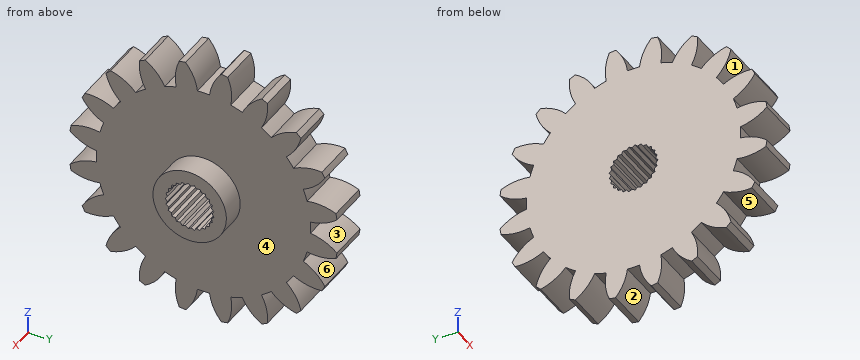
from build123d import *

# Parameters (mm, degrees)
BASPROSKE_W         = 5
BASPROSKE_H         = 16.5
TOOTHCUT_DEPTH      = 24.864199128
TEETHCUTS_COUNT     = 20
TEETHCUTS_ANGLE     = 342
BORSKE_R            = 2.5
BORE_DEPTH          = 50.0000508
BOSS_EXTRUDE1_START = 3
SKETCH1_R           = 4.5
SKETCH1_R_2         = 2.5
BOSS_EXTRUDE1_DEPTH = 3
SKETCH2_R           = 2.75
SKETCH2_R_2         = 2.5
CUT_EXTRUDE1_DEPTH  = 25.472631648
CIRPATTERN1_COUNT   = 25


with BuildPart() as part:
    # BasProSke → Base-Revolve (revolve)
    with BuildSketch(Plane(origin=(0, 0, 0), x_dir=(1, 0, 0), z_dir=(0, 1, 0)), mode=Mode.PRIVATE) as base_revolve_sk:
        with Locations((2.5, 8.25)):
            Rectangle(BASPROSKE_W, BASPROSKE_H)
    revolve(base_revolve_sk.sketch.rotate(Axis((-10, 0, 0), (1, 0, 0)), 180), axis=Axis((-10, 0, 0), (1, 0, 0)))

    # TooCutSke → ToothCut (cut, through all)
    with BuildSketch(Plane(origin=(0, 0, 0), x_dir=(0, 0, -1), z_dir=(1, 0, 0))):
        with BuildLine():
            ThreePointArc((0.74381438, 13.102904875), (0, 13.124), (-0.74381438, 13.102904875))
            ThreePointArc((-0.74381438, 13.102904875), (-1.226473103, 14.852072512), (-2.209965745, 16.376962373))
            ThreePointArc((-2.209965745, 16.376962373), (0, 16.5254), (2.209965745, 16.376962373))
            ThreePointArc((2.209965745, 16.376962373), (1.226473103, 14.852072512), (0.74381438, 13.102904875))
        make_face()
    toothcut = extrude(amount=TOOTHCUT_DEPTH, mode=Mode.SUBTRACT)

    # TeethCuts: ToothCut ×20 about axis
    teethcuts_axis = Axis((-10, 0, 0), (1, 0, 0))
    for i in range(1, TEETHCUTS_COUNT):
        add(toothcut.rotate(teethcuts_axis, i * TEETHCUTS_ANGLE / (TEETHCUTS_COUNT - 1)), mode=Mode.SUBTRACT)

    # BorSke → Bore (cut, symmetric)
    with BuildSketch(Plane(origin=(0, 0, 0), x_dir=(0, 0, -1), z_dir=(1, 0, 0))):
        with Locations(Location((0, 0, 0), (0, 0, 180))):
            Circle(BORSKE_R)
    extrude(amount=BORE_DEPTH, both=True, mode=Mode.SUBTRACT)

    # Sketch1 → Boss-Extrude1 (add)
    with BuildSketch(Plane(origin=(5, 0, 0), x_dir=(0, 0, -1), z_dir=(1, 0, 0)).offset(BOSS_EXTRUDE1_START)):
        with Locations(Location((0, 0, 0), (0, 0, 180))):
            Circle(SKETCH1_R)
        Circle(SKETCH1_R_2, mode=Mode.SUBTRACT)
    extrude(amount=-BOSS_EXTRUDE1_DEPTH)

    # Sketch2 → Cut-Extrude1 (cut, through all)
    # profile 1 of 2: a face of its own
    with BuildSketch(Plane(origin=(8, 0, 0), x_dir=(0, 0, -1), z_dir=(1, 0, 0))):
        with BuildLine():
            ThreePointArc((0.344666392, -2.728315429), (0, -2.75), (-0.344666392, -2.728315429))
            Line((-0.344666392, -2.728315429), (0, -3))
            Line((0, -3), (0.344666392, -2.728315429))
        make_face()
    # profile 2 of 2: a face of its own
    with BuildSketch(Plane(origin=(8, 0, 0), x_dir=(0, 0, -1), z_dir=(1, 0, 0))):
        Circle(SKETCH2_R)
        Circle(SKETCH2_R_2, mode=Mode.SUBTRACT)
    cut_extrude1 = extrude(amount=-CUT_EXTRUDE1_DEPTH, mode=Mode.SUBTRACT)

    # CirPattern1: Cut-Extrude1 ×25 about axis
    cirpattern1_axis = Axis((0, 0, 0), (1, 0, 0))
    for i in range(1, CIRPATTERN1_COUNT):
        add(cut_extrude1.rotate(cirpattern1_axis, i * 360 / CIRPATTERN1_COUNT), mode=Mode.SUBTRACT)


solid = part.part
Here's how the part is built. I have some questions about the finished solid (model axes, mm). Face numbers are marked on the shaded views. A direction names the side the tool comes from. Give positions to 0.01 mm unless a question says otherwise; leave off trailing zeros. Write each loop counter-clockwise with the first axis right and the second up, starting at its lowest first coordinate (ties: lowest second). Pieces come first, ordered by that corner, then holes. Notation, with made-up numbers: (-22.75, -32) -> (-3.75, -32) arc R11 ccw to (-3.75, -22) -> close; hole circle Ø6 at (-36.5, -4). An arc over 180 degrees is marked (long way). Use one line per item in the form item = value. Start each with the question number.
1. If I drill on L1, parallel to Z at x = 3.75, y = 11.5; L2, parallel to Y at x = 1.75, z = 14; L3, parallel to X at y = -8, z = 5, over which ranges is the centre line in solid material (lowest first)?
2. Will these pins go through, and if not, where does the flat tip stop? pin 1 Ø3 at (y, z) = (-4.5, 8.5) entering from +X; pin 2 Ø10 at (y, z) = (-1, -5.5) entering from +X; pin 3 Ø3 at (x, z) = (2, -6) entering from -Y; pin 4 Ø1 at (x, y) = (4.5, -10.5) entering from -Z.
3. Imagine slicing it at A-A on y = 13.5. List the corners of the cut face in (x, z) for me, plus the area to 3 significant figures.
4. On a 3-axis mill with a long thin cutter (end or side, diameter ignored), from which of +Z, -Z, +X, -X, +Y, -Y can I reach the whole of each face in a straight line? I mean the marked faces 4, 5 and 6. Say none if no direction works.
5. Imagine slicing it at B-B on y = -6. List the corners of the cut face in (x, z) for me.
6. Thinking about a two-plate mould opening in Y: for the marked faces 1, 2 and 3, which applies, +Y half, -Y half, draft (parallel to the pull), parting line (faces both ways), or undercut?
7. Imagine slicing it at C-C on z = 6.5. List the corners of the cut face in (x, y) for me.
Entries:
q1.L1 = -11.83 to -10.11, -7.33 to 7.33, 10.11 to 11.83
q1.L2 = -7.87 to -6, -3.46 to -0.92, 0.92 to 3.46, 6 to 7.87
q1.L3 = 0 to 5
q2.pin_1 = 5
q2.pin_2 = 8
q2.pin_3 = -14.88
q2.pin_4 = -11.84
q3.outline = (0, -7.85) -> (5, -7.85) -> (5, -5.55) -> (0, -5.55) -> close; (0, -3.45) -> (5, -3.45) -> (5, -0.8) -> (0, -0.8) -> close; (0, 0.8) -> (5, 0.8) -> (5, 3.45) -> (0, 3.45) -> close; (0, 5.55) -> (5, 5.55) -> (5, 7.85) -> (0, 7.85) -> close
q3.area = 49.4 mm²
q4.face_4 = +X
q4.face_5 = +X, -X
q4.face_6 = +X, -X, +Y
q5.outline = (0, -14) -> (5, -14) -> (5, 14) -> (0, 14) -> close
q6.face_1 = -Y half
q6.face_2 = undercut
q6.face_3 = +Y half
q7.outline = (0, -14.44) -> (5, -14.44) -> (5, 14.44) -> (0, 14.44) -> close
